Verification items for the finished model (mm, model axes). A direction names the side the tool comes from. Coordinates: 2 decimals unless noted, no trailing zeros. Loops run counter-clockwise (first coordinate to the right, second up) from the corner with the lowest first, then second, coordinate; pieces in that order, holes last. Notation, with made-up numbers: (-9, -3.5) -> (30, -3.5) arc R25 cw to (30, 34.5) -> close; hole circle Ø4 at (60, 26). An arc over 180 degrees is marked (long way). Answer as a JSON object with one key per item and string values. Group by question number.
Q1. Set-up check for faces 1 (the flat face through (-42, 2.5, 10)), 2 (the flat face through (-1, -7.5, 3)), 3 (the cylindrical face through (-30.25, 0.95, 10.06)), 4 (the flat face through (-14, -5, 15)), 5 (the flat face through (57.5, 0, 10)): record each of +Z, -Z, +X, -X, +Y, -Y from which the full face is reachable in a straight line by a thin tool's end or side.
Q2. Cross-section at D-D on z = 18. Record the boundary of the cut face in (x, y).
Q3. Cross-section at C-C on x = -49.5. Record the boundary of the cut face in (y, z).
Q4. Gauge pin test, flat ends, axial feed: pin 1 Ø5.5 at (x, z) = (12, 12.5) entering from -Y; pin 2 Ø1 at (x, z) = (-14.5, 7) entering from -Y; pin 3 Ø6 at (x, z) = (-41.5, 13) entering from +Y. Record the tip position at first contact, or that the pin passes through.
Q5. Release check for a two-part mould opening along Z. For faces 6 (the cylindrical face through (9.492, 2.422, 7.381)), 7 (the flat face through (-35.5, 4, 10)) record: released by +Z, released by -Z, zero draft, split by the parting line, or undercut.
Q6. Cross-section at B-B on y = 1. Record the boundary of the cut face in (x, z), and give its area (3 significant figures).
Q7. Cross-section at A-A on x = 30.5. Record the boundary of the cut face in (y, z).
Q8. Scan lines: L1, parallel to X at y = -4.8, z = 10; L2, parallel to Z at x = 20.5, y = -4.5; L3, parallel to Z at x = -4.5, y = -6.25. Record each from-to range of solid material in increasing order.
```python
from build123d import *

# Parameters (mm, degrees)
SKETCH_1_W                 = 115
SKETCH_1_H                 = 15
EXTRUDE_1_DEPTH            = 20
SKETCH_2_W                 = 12
SKETCH_2_H                 = 20
CUT_EXTRUDE_1_DEPTH        = 5
SKETCH_3_W                 = 40
SKETCH_3_H                 = 20
CUT_EXTRUDE_2_DEPTH        = 3
HOLE_START                 = -7.5
HOLE_WIZARD_M6_1_OUTLINE_R = 2.5
HOLE_WIZARD_M6_1_DEPTH     = 10
CUT_EXTRUDE_3_DEPTH        = 5
CUT_EXTRUDE_4_DEPTH        = 20
HOLE_WIZARD_3_D            = 6.6
HOLE_WIZARD_3_DEPTH        = 15
HOLE_WIZARD_3_CBORE_D      = 11
HOLE_WIZARD_3_CBORE_DEPTH  = 4.7
HOLE_WIZARD_3_TIP          = 1.982840043
HOLE_WIZARD_M5_1_D         = 4.2
HOLE_WIZARD_M5_1_DEPTH     = 12.4
HOLE_WIZARD_M5_1_TIP       = 1.2618073


# Read off the part's stored shape, not the designer's step: M6 螺纹孔1
with BuildPart() as part:
    # 草图1 → 凸台-拉伸1 (new body)
    with BuildSketch(Plane.XY):
        Rectangle(SKETCH_1_W, SKETCH_1_H)
    extrude(amount=EXTRUDE_1_DEPTH)

    # 草图2 → 切除-拉伸1 (cut)
    with BuildSketch(Plane(origin=(0, 7.5, 0), x_dir=(1, 0, 0), z_dir=(0, 1, 0))):
        with Locations((-41.5, -10)):
            Rectangle(SKETCH_2_W, SKETCH_2_H)
    extrude(amount=-CUT_EXTRUDE_1_DEPTH, mode=Mode.SUBTRACT)

    # 草图3 → 切除-拉伸2 (cut)
    with BuildSketch(Plane(origin=(0, 7.5, 0), x_dir=(1, 0, 0), z_dir=(0, 1, 0))):
        with Locations((-15.5, -10)):
            Rectangle(SKETCH_3_W, SKETCH_3_H)
    extrude(amount=-CUT_EXTRUDE_2_DEPTH, mode=Mode.SUBTRACT)

    # M6 螺纹孔1 outline → M6 螺纹孔1 (cut)
    with BuildSketch(Plane(origin=(0, 0, 0), x_dir=(1, 0, 0), z_dir=(0, 1, 0)).offset(HOLE_START)):
        with Locations((-49.5, -10)):
            Circle(HOLE_WIZARD_M6_1_OUTLINE_R)
    extrude(amount=HOLE_WIZARD_M6_1_DEPTH, mode=Mode.SUBTRACT)

    # Hole Wizard M6 _1 2 outline → Hole Wizard M6 _1 2 (revolve, cut)
    with BuildSketch(Plane(origin=(20.5, 0, 10), x_dir=(1, 0, 0), z_dir=(0, 0, 1))):
        Polygon((2.5, 2.5), (0, 4.002151548), (0, -7.5), (2.5, -7.5), align=None)
    revolve(axis=Axis((20.5, 0, 10), (0, 1, 0)), mode=Mode.SUBTRACT)

    # 草图6 → 切除-拉伸3 (cut)
    with BuildSketch(Plane.XZ.offset(7.5)):
        with BuildLine():
            Line((-27.5, 15), (0.5, 15))
            ThreePointArc((0.5, 15), (5.5, 10), (0.5, 5))
            Line((0.5, 5), (-27.5, 5))
            ThreePointArc((-27.5, 5), (-32.5, 10), (-27.5, 15))
        make_face()
    extrude(amount=-CUT_EXTRUDE_3_DEPTH, mode=Mode.SUBTRACT)

    # 草图7 → 切除-拉伸4 (cut)
    with BuildSketch(Plane.XZ.offset(2.5)):
        with BuildLine():
            Line((-27.5, 7.25), (0.5, 7.25))
            ThreePointArc((0.5, 7.25), (3.25, 10), (0.5, 12.75))
            Line((0.5, 12.75), (-27.5, 12.75))
            ThreePointArc((-27.5, 12.75), (-30.25, 10), (-27.5, 7.25))
        make_face()
    extrude(amount=-CUT_EXTRUDE_4_DEPTH, mode=Mode.SUBTRACT)

    # 打孔尺寸(%根据)内六角花形圆柱头螺钉3
    with Locations(Plane(origin=(11.5, -7.5, 10), x_dir=(0, 0, -1), z_dir=(0, -1, 0))):
        with Locations((0, 0), (0, 19)):
            CounterBoreHole(HOLE_WIZARD_3_D / 2, HOLE_WIZARD_3_CBORE_D / 2, HOLE_WIZARD_3_CBORE_DEPTH, depth=HOLE_WIZARD_3_DEPTH)
            with Locations((0, 0, -(HOLE_WIZARD_3_DEPTH + HOLE_WIZARD_3_TIP / 2))):  # 118° drill point
                Cone(0, HOLE_WIZARD_3_D / 2, HOLE_WIZARD_3_TIP, mode=Mode.SUBTRACT)

    # M5 螺纹孔1
    with Locations(Plane(origin=(-57.5, 4.5, 10), x_dir=(0, 0, -1), z_dir=(-1, 0, 0))):
        with Locations((0, 0)):
            Hole(HOLE_WIZARD_M5_1_D / 2, depth=HOLE_WIZARD_M5_1_DEPTH)
            with Locations((0, 0, -(HOLE_WIZARD_M5_1_DEPTH + HOLE_WIZARD_M5_1_TIP / 2))):  # 118° drill point
                Cone(0, HOLE_WIZARD_M5_1_D / 2, HOLE_WIZARD_M5_1_TIP, mode=Mode.SUBTRACT)


solid = part.part
```
Computed values:
{
 "1": {"face 1": "+Z, -Z, +Y", "face 2": "+Z, -Z, +X, -X, -Y", "face 3": "+Y, -Y", "face 4": "-Y", "face 5": "+Z, -Z, +X, +Y, -Y"},
 "2": {"outline": "(-57.5, -7.5) -> (57.5, -7.5) -> (57.5, 7.5) -> (4.5, 7.5) -> (4.5, 4.5) -> (-35.5, 4.5) -> (-35.5, 2.5) -> (-47.5, 2.5) -> (-47.5, 7.5) -> (-57.5, 7.5) -> close"},
 "3": {"outline": "(-7.5, 0) -> (7.5, 0) -> (7.5, 20) -> (-7.5, 20) -> (-7.5, 12.5) -> (2.5, 12.5) -> (2.5, 10.64) arc R2.1 cw (long way) to (2.5, 9.36) -> (2.5, 7.5) -> (-7.5, 7.5) -> close"},
 "4": {"pin 1": "stops at y = -2.8", "pin 2": "stops at y = -2.5", "pin 3": "stops at y = 2.5"},
 "5": {"face 6": "undercut", "face 7": "zero draft"},
 "6": {"outline": "(-57.5, 0) -> (57.5, 0) -> (57.5, 20) -> (-57.5, 20) -> close; hole circle Ø5 at (-49.5, 10); hole (-27.5, 7.25) -> (0.5, 7.25) arc R2.75 ccw to (0.5, 12.75) -> (-27.5, 12.75) arc R2.75 ccw to start; hole circle Ø6.6 at (11.5, 10); hole circle Ø5 at (20.5, 10); hole circle Ø6.6 at (30.5, 10)", "area": "2,010 mm²"},
 "7": {"outline": "(-7.5, 0) -> (7.5, 0) -> (7.5, 6.7) -> (-2.8, 6.7) -> (-2.8, 4.5) -> (-7.5, 4.5) -> close; (-7.5, 15.5) -> (-2.8, 15.5) -> (-2.8, 13.3) -> (7.5, 13.3) -> (7.5, 20) -> (-7.5, 20) -> close"},
 "8": {"L1": "x = -57.5 to -52, -47 to -32.5, 5.5 to 6, 17 to 18, 23 to 25, 36 to 57.5", "L2": "z = 0 to 7.5, 12.5 to 20", "L3": "z = 0 to 5, 15 to 20"}
}
